Geometry: final body of the model. Coordinates: model frame, mm. A direction names the side the tool comes from. Give positions to 0.01 mm unless a question says otherwise; leave off trailing zeros. Order: outer loops, then holes, each group sorted by start corner. A loop starts at its lowest first (then second) coordinate and runs counter-clockwise, first axis right, second up. Notation, with made-up numbers: (6.25, 4.25) - (57.25, 4.25) arc R17 ccw to (57.25, 14.25) - close; hole circle Ø7 at (88.5, 72). An arc over 180 degrees is marked (long way). Use one line per item in the form item = value.
from build123d import *

# Parameters (mm, degrees)
SKETCH1_W            = 39.5
SKETCH1_H            = 14.5
SKETCH1_W_2          = 15
SKETCH1_H_2          = 9
BOSS_EXTRUDE1_DEPTH  = 3
FILLET1_R            = 4
M4_CLEARANCE_HOLE1_D = 4.8
CHAMFER1_SIZE        = 0.5


with BuildPart() as part:
    # Sketch1 → Boss-Extrude1 (new body)
    with BuildSketch(Plane(origin=(0, 0, 0), x_dir=(1, 0, 0), z_dir=(0, 1, 0))):
        Rectangle(SKETCH1_W, SKETCH1_H)
        Rectangle(SKETCH1_W_2, SKETCH1_H_2, mode=Mode.SUBTRACT)
    extrude(amount=BOSS_EXTRUDE1_DEPTH)

    # Fillet1
    fillet1_edges = [part.edges().sort_by_distance(p)[0] for p in [
        (19.75, 1.5, 7.25),
        (-19.75, 1.5, 7.25),
        (-19.75, 1.5, -7.25),
        (19.75, 1.5, -7.25),
    ]]
    fillet(fillet1_edges, radius=FILLET1_R)

    # M4 Clearance Hole1 (through all)
    with Locations(Plane(origin=(0, 3, 0), x_dir=(1, 0, 0), z_dir=(0, 1, 0))):
        with Locations((-15.5, 0), (15.5, 0)):
            Hole(M4_CLEARANCE_HOLE1_D / 2)

    # Chamfer1
    chamfer1_edges = [part.edges().sort_by_distance(p)[0] for p in [
        (19.75, 0, 0),
        (19.75, 3, 0),
        (0, 0, 7.25),
        (-19.75, 0, 0),
        (0, 0, -7.25),
        (-18.578427125, 0, -6.078427125),
        (-18.578427125, 0, 6.078427125),
        (18.578427125, 0, -6.078427125),
        (18.578427125, 0, 6.078427125),
        (0, 3, 7.25),
        (0, 3, -7.25),
        (-19.75, 3, 0),
        (-18.578427125, 3, -6.078427125),
        (-18.578427125, 3, 6.078427125),
        (18.578427125, 3, -6.078427125),
        (18.578427125, 3, 6.078427125),
    ]]
    chamfer(chamfer1_edges, length=CHAMFER1_SIZE)


solid = part.part
(1) Cut plane C-C on z = 0. Output: boundary loops of the cut face in (x, y).
Computed values:
outline = (-19.75, 0.5) - (-19.25, 0) - (-17.9, 0) - (-17.9, 3) - (-19.25, 3) - (-19.75, 2.5) - close; (-13.1, 0) - (-7.5, 0) - (-7.5, 3) - (-13.1, 3) - close; (7.5, 0) - (13.1, 0) - (13.1, 3) - (7.5, 3) - close; (17.9, 0) - (19.25, 0) - (19.75, 0.5) - (19.75, 2.5) - (19.25, 3) - (17.9, 3) - close
(2) Cut plane A-A on x = 1. Output: boundary loops of the cut face in (y, z), plus the area to 3 significant figures.
Computed values:
outline = (0, -6.75) - (0.5, -7.25) - (2.5, -7.25) - (3, -6.75) - (3, -4.5) - (0, -4.5) - close; (0, 4.5) - (3, 4.5) - (3, 6.75) - (2.5, 7.25) - (0.5, 7.25) - (0, 6.75) - close
area = 16.0 mm²
(3) Pull-direction query (Y, two-part tool) for faces 3 (the face through (-7.5, 1, 0)), 4 (the face through (-18.3, 2.86, -5.85)), 5 (the face through (-18.35, 0.14, 5.8)); classes: released by +Y, released by -Y, zero draft, split by the parting line, or undercut.
Computed values:
face_3 = zero draft
face_4 = released by +Y
face_5 = released by -Y
(4) Cut plane B-B on y = 1.25. Output: boundary loops of the cut face in (x, z).
Computed values:
outline = (-19.75, -3.25) arc R4 ccw to (-15.75, -7.25) - (15.75, -7.25) arc R4 ccw to (19.75, -3.25) - (19.75, 3.25) arc R4 ccw to (15.75, 7.25) - (-15.75, 7.25) arc R4 ccw to (-19.75, 3.25) - close; hole circle Ø4.8 at (-15.5, 0); hole (-7.5, -4.5) - (7.5, -4.5) - (7.5, 4.5) - (-7.5, 4.5) - close; hole circle Ø4.8 at (15.5, 0)
(5) Cut plane D-D on z = -1.5. Output: boundary loops of the cut face in (x, y).
Computed values:
outline = (-19.75, 0.5) - (-19.25, 0) - (-17.37, 0) - (-17.37, 3) - (-19.25, 3) - (-19.75, 2.5) - close; (-13.63, 0) - (-7.5, 0) - (-7.5, 3) - (-13.63, 3) - close; (7.5, 0) - (13.63, 0) - (13.63, 3) - (7.5, 3) - close; (17.37, 0) - (19.25, 0) - (19.75, 0.5) - (19.75, 2.5) - (19.25, 3) - (17.37, 3) - close
(6) Contact query for a flat-ended pin moving along its axis: pin 1 Ø3 at (x, z) = (-15.5, 0) entering from -Y. Output: stop coordinate, or through.
Computed values:
pin_1 = through
(7) Reachability of faces 1 (the face through (-19.75, 1, 0)), 2 (the face through (0, 1, 4.5)) from +Z, -Z, +X, -X, +Y, -Y: full face, straight path, thin tool, end or side. Return the list, or none.
Computed values:
face_1 = +Z, -Z, -X, +Y, -Y
face_2 = +Y, -Y
(8) Ray query, line 1 along Z through (x, y) = (15.5, 0.7); line 2 along X through (y, z) = (1.4, -1.5); line 3 along X through (y, z) = (1.8, 0.5). Return the intervals inside material, ascending.
Computed values:
line_1 = -7.25 to -2.4, 2.4 to 7.25
line_2 = -19.75 to -17.37, -13.63 to -7.5, 7.5 to 13.63, 17.37 to 19.75
line_3 = -19.75 to -17.85, -13.15 to -7.5, 7.5 to 13.15, 17.85 to 19.75
